The listing builds one solid part. Answer for the finished solid, in the listing's coordinates (mm). Face numbers are marked on the shaded views. A direction names the side the tool comes from. Round coordinates to 2 decimals unless told otherwise and drop trailing zeros. Write each loop counter-clockwise with the first axis right and the second up, starting at its lowest first coordinate (ties: lowest second). Pieces come first, ordered by that corner, then holes. Notation, with made-up numbers: (-37.75, 7) - (-22.75, 7) arc R25 cw to (-22.75, 35) - close; hole circle Ø4 at (13, 18). An arc over 180 degrees is marked (long way). Answer as CSV lines item,"result". Start each with the question number.
Item 1: For a pull along Y with two mould halves and no side action, classify the marked faces 4, 5, 6 and 7 as pulls with the +Y half, pulls with the -Y half, needs draft (parallel to the pull), parting line crosses it, or undercut.
Item 2: Straight lines are drawn through the part: line 1 along Y through (x, z) = (0, 9); line 2 along Z through (x, y) = (-12, -7); line 3 along Y through (x, z) = (-16, 24). For each, find the intervals that lie inside material, in ascending order. Write a range as [from, to].
Item 3: A cutting plane is placed at B-B on y = 50. Determine the outline of the cut face in (x, z), and give its area (3 significant figures).
Item 4: A cutting plane is placed at C-C on y = -16. Determine the outline of the cut face in (x, z), and give its area (3 significant figures).
Item 5: Which of the six approach directions +Z, -Z, +X, -X, +Y, -Y give full straight-line access (tool end or side, diameter ignored) to the marked faces 1, 2 and 3?
Item 6: A cutting plane is placed at A-A on x = 0. Determine the outline of the cut face in (y, z), and give its area (3 significant figures).
Item 7: A cutting plane is placed at D-D on z = 49.5. Determine the outline of the cut face in (x, y).
Item 8: Flat-ended cylindrical pins translate along their axes: pin 1 (10.5 mm diameter, centred on x = 17.5, y = -20, fed in from +Z); pin 2 (5.5 mm diameter, centred on y = -23, z = 45, fed in from +X); pin 3 (10 mm diameter, centred on x = -1.5, y = 1, fed in from +Z). Find the tip coordinate at first contact, or state that the pin passes through.
```python
from build123d import *

# Parameters (mm, degrees)
F1_DEPTH = 19.05
F2_W     = 44.5915646851
F2_H     = 22.1683774143
F3_DEPTH = 38.1
F4_W     = 21.1491398513
F4_H     = 22.1683774143
F5_DEPTH = 19.05
F6_R     = 19.9367778841
F7_DEPTH = 25.4


with BuildPart() as f1:
    # F0 (on Top) → F1 (new body)
    with BuildSketch(Plane.XY):
        with BuildLine():
            ThreePointArc((32.8703522682, 32.8703522682), (0, 65.7407045364), (-32.8703522682, 32.8703522682))
            Line((-32.8703522682, 32.8703522682), (32.8703522682, 32.8703522682))
        make_face()
        with BuildLine():
            ThreePointArc((32.8703522682, 32.8703522682), (0, 0), (-32.8703522682, 32.8703522682))
            Line((-32.8703522682, 32.8703522682), (-32.8703522682, -32.8703522682))
            Line((-32.8703522682, -32.8703522682), (32.8703522682, -32.8703522682))
            Line((32.8703522682, -32.8703522682), (32.8703522682, 32.8703522682))
        make_face()
        with BuildLine():
            Line((32.8703522682, 32.8703522682), (-32.8703522682, 32.8703522682))
            ThreePointArc((-32.8703522682, 32.8703522682), (0, 0), (32.8703522682, 32.8703522682))
        make_face()
    extrude(amount=F1_DEPTH)

    # F2 (on face) → F3 (join)
    with BuildSketch(Plane.XY.offset(19.05)):
        with Locations((-10.5745699257, -21.786163561)):
            Rectangle(F2_W, F2_H)
    extrude(amount=F3_DEPTH)

    # F4 (on face) → F5 (join)
    with BuildSketch(Plane.XY.offset(19.05)):
        with Locations((22.2957823426, -21.786163561)):
            Rectangle(F4_W, F4_H)
    extrude(amount=F5_DEPTH)

    # F6 (on face) → F7 (cut)
    with BuildSketch(Plane.XY.offset(19.05)):
        with Locations((0, 32.8703522682)):
            Circle(F6_R)
    extrude(amount=-F7_DEPTH, mode=Mode.SUBTRACT)


solid = f1.part
```
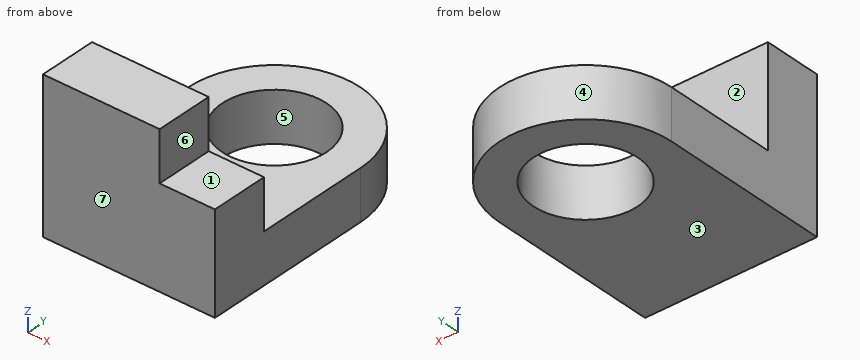
Geometry says:
1,face 4,"pulls with the +Y half"
1,face 5,"undercut"
1,face 6,"needs draft"
1,face 7,"pulls with the -Y half"
2,line 1,"y = [-32.87, 12.93], [52.81, 65.74]"
2,line 2,"z = [0, 19.05]"
2,line 3,"y = [-32.87, -10.7]"
3,outline,"(-28.05, 0) - (-10.2, 0) - (-10.2, 19.05) - (-28.05, 19.05) - close; (10.2, 0) - (28.05, 0) - (28.05, 19.05) - (10.2, 19.05) - close"
3,area,"680 mm^2"
4,outline,"(-32.87, 0) - (32.87, 0) - (32.87, 38.1) - (11.72, 38.1) - (11.72, 57.15) - (-32.87, 57.15) - close"
4,area,"3,350 mm^2"
5,face 1,"+Z, +X, +Y, -Y"
5,face 2,"+Z, +X, -X, +Y"
5,face 3,"-Z, +X, -X, +Y, -Y"
6,outline,"(-32.87, 0) - (12.93, 0) - (12.93, 19.05) - (-10.7, 19.05) - (-10.7, 57.15) - (-32.87, 57.15) - close; (52.81, 0) - (65.74, 0) - (65.74, 19.05) - (52.81, 19.05) - close"
6,area,"1,960 mm^2"
7,outline,"(-32.87, -32.87) - (11.72, -32.87) - (11.72, -10.7) - (-32.87, -10.7) - close"
8,pin 1,"stops at z = 38.1"
8,pin 2,"stops at x = 11.72"
8,pin 3,"stops at z = 19.05"
